CAD build for the part. Positions are in the model's coordinates, mm. Face numbers are marked on the shaded views. A direction names the side the tool comes from. Round coordinates to 2 decimals unless told otherwise and drop trailing zeros. Order: outer loops, then holes, each group sorted by start corner. A loop starts at its lowest first (then second) coordinate and runs counter-clockwise, first axis right, second up. Notation, with made-up numbers: M 75.5,89 L 110.5,89 A25 ccw 110.5,125 Z; hole C 20.25,-34.75 d6. An arc over 180 degrees is marked long. Answer as a JSON object with one key per item and string values.
```python
from build123d import *

# Parameters (mm, degrees)
CYLINDER024_R             = 13
CYLINDER024_DEPTH         = 45
CYLINDER026_R             = 1.95
CYLINDER026_DEPTH         = 10
BOX002_W                  = 21.4
BOX002_H                  = 3.9
BOX002_DEPTH              = 10
FUSION013_PLACEMENT_ANGLE = 90
ARRAY011_COUNT            = 3
CYLINDER028_R             = 2.2
CYLINDER028_DEPTH         = 5
ARRAY013_X_COUNT          = 2
ARRAY013_X_PITCH          = 70
BOX003_W                  = 70
BOX003_H                  = 12
BOX003_DEPTH              = 5
BOX007_W                  = 60
BOX007_H                  = 3
BOX007_DEPTH              = 5
FILLET003_R               = 3
CYLINDER027_R             = 6
CYLINDER027_DEPTH         = 5
ARRAY012_X_COUNT          = 2
ARRAY012_X_PITCH          = 70
CYLINDER025_R             = 16
CYLINDER025_DEPTH         = 45
FUSION016_PLACEMENT_ANGLE = 25
FILLET005_R               = 2


with BuildPart() as internal_cylinder:
    # Cylinder024 → Cylinder024 (new body)
    with BuildSketch(Plane.XY.offset(5)):
        Circle(CYLINDER024_R)
    extrude(amount=CYLINDER024_DEPTH)


with BuildPart() as hole_side001:
    # Cylinder026 → Cylinder026 (new body)
    with BuildSketch(Plane(origin=(21.4, 0, 0), x_dir=(1, 0, 0), z_dir=(0, 0, 1))):
        Circle(CYLINDER026_R)
    extrude(amount=CYLINDER026_DEPTH)


with BuildPart() as middle_hole_fusion:
    # Box002 → Box002 (new body)
    with BuildSketch(Plane(origin=(0, -1.95, 0), x_dir=(1, 0, 0), z_dir=(0, 0, 1))):
        with Locations((10.7, 1.95)):
            Rectangle(BOX002_W, BOX002_H)
    extrude(amount=BOX002_DEPTH)

    # Fusion013: union hole side001
    add(hole_side001.part)


with BuildPart() as middle_hole_fusion_1:
    # Fusion013 placement: moved
    add(middle_hole_fusion.part.moved(Location((-6, 0, 0))).rotate(Axis((-6, 0, 0), (0, -1, 0)), FUSION013_PLACEMENT_ANGLE))

    # Array011: middle hole fusion ×3 about axis
    array011_axis = Axis((0, 0, 0), (0, 0, 1))


with BuildPart() as middle_hole_fusion_2:
    add(middle_hole_fusion_1.part)
    for i in range(1, ARRAY011_COUNT):
        add(middle_hole_fusion_1.part.rotate(array011_axis, i * 360 / ARRAY011_COUNT))


with BuildPart() as middle_hole_fusion_3:
    # Array011 placement: moved
    add(middle_hole_fusion_2.part.moved(Location((0, 0, 5))))

    # Fusion014: union internal cylinder
    add(internal_cylinder.part)


with BuildPart() as spring_plate_end_array001:
    # Cylinder028 → Cylinder028 (new body)
    with BuildSketch(Plane.XY):
        Circle(CYLINDER028_R)
    extrude(amount=CYLINDER028_DEPTH)

    # Array013 X: spring plate end array001 ×2


with BuildPart() as spring_plate_end_array001_1:
    add(spring_plate_end_array001.part)
    with Locations(*[(i * ARRAY013_X_PITCH, 0, 0) for i in range(1, ARRAY013_X_COUNT)]):
        add(spring_plate_end_array001.part)


with BuildPart() as spring_plate_cube:
    # Box003 → Box003 (new body)
    with BuildSketch(Plane(origin=(0, -6, 0), x_dir=(1, 0, 0), z_dir=(0, 0, 1))):
        with Locations((35, 6)):
            Rectangle(BOX003_W, BOX003_H)
    extrude(amount=BOX003_DEPTH)


with BuildPart() as fillet003:
    # Box007 → Box007 (new body)
    with BuildSketch(Plane(origin=(5, -1.5, -5), x_dir=(1, 0, 0), z_dir=(0, 0, 1))):
        with Locations((30, 1.5)):
            Rectangle(BOX007_W, BOX007_H)
    extrude(amount=BOX007_DEPTH)

    # Fillet003
    fillet003_edges = [fillet003.edges().sort_by_distance(p)[0] for p in [
        (5, 0, -5),
        (65, 0, -5),
    ]]
    fillet(fillet003_edges, radius=FILLET003_R)


with BuildPart() as spring_attachment_plate:
    # Cylinder027 → Cylinder027 (new body)
    with BuildSketch(Plane.XY):
        Circle(CYLINDER027_R)
    extrude(amount=CYLINDER027_DEPTH)

    # Array012 X: spring attachment plate ×2


with BuildPart() as spring_attachment_plate_1:
    add(spring_attachment_plate.part)
    with Locations(*[(i * ARRAY012_X_PITCH, 0, 0) for i in range(1, ARRAY012_X_COUNT)]):
        add(spring_attachment_plate.part)

    # Fusion015: union spring plate cube, Fillet003
    add(spring_plate_cube.part)
    add(fillet003.part)

    # Cut009: cut spring plate end array001
    add(spring_plate_end_array001_1.part, mode=Mode.SUBTRACT)


with BuildPart() as spring_attachment_plate_2:
    # Cut009 placement: moved
    add(spring_attachment_plate_1.part.moved(Location((-35, 0, 45))))


with BuildPart() as middle_cut_fillet:
    # Cylinder025 → Cylinder025 (new body)
    with BuildSketch(Plane.XY.offset(5)):
        Circle(CYLINDER025_R)
    extrude(amount=CYLINDER025_DEPTH)

    # Fusion016: union spring attachment plate
    add(spring_attachment_plate_2.part)


with BuildPart() as middle_cut_fillet_1:
    # Fusion016 placement: moved
    add(middle_cut_fillet.part.rotate(Axis((0, 0, 0), (0, 0, 1)), FUSION016_PLACEMENT_ANGLE))

    # Cut008: cut middle hole fusion
    add(middle_hole_fusion_3.part, mode=Mode.SUBTRACT)

    # Fillet005
    fillet005_edges = [middle_cut_fillet_1.edges().sort_by_distance(p)[0] for p in [
        (8.872161, -11.467033, 5),
        (8.872161, 11.467033, 5),
        (5.494662, -13.417033, 5),
        (-14.366823, -1.95, 5),
        (-14.366823, 1.95, 5),
        (5.494662, 13.417033, 5),
    ]]
    fillet(fillet005_edges, radius=FILLET005_R)


solid = middle_cut_fillet_1.part
```
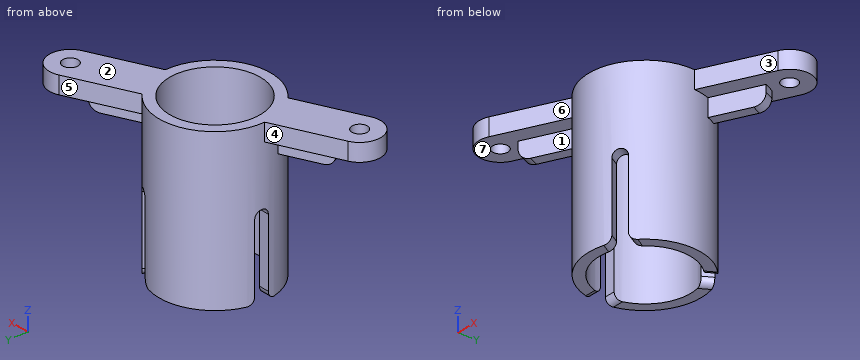
Item 1: Saw through at C-C on x = 0. List the corners of the cut face in (y, z).
Worked answers:
{"outline": "M -16,5 L -13,5 L -13,50 L -16,50 Z; M 13,5 L 16,5 L 16,50 L 13,50 Z"}
Item 2: Saw through at D-D on x = -17.5. List the corners of the cut face in (y, z), and give its area (3 significant figures).
Worked answers:
{"outline": "M -14.78,45 L -9.82,45 L -9.82,40 L -6.51,40 L -6.51,45 L -1.54,45 L -1.54,50 L -14.78,50 Z", "area": "82.8 mm2"}
Item 3: Saw through at B-B on y = 0. List the corners of the cut face in (x, z).
Worked answers:
{"outline": "M -16,28.35 L -13,28.35 L -13,50 L -16,50 Z; M 13,5 L 16,5 L 16,50 L 13,50 Z"}
Item 4: Saw through at A-A on z = 23.5. List the corners of the cut face in (x, y).
Worked answers:
{"outline": "M -15.88,-1.95 A16 ccw 6.25,-14.73 L 4.74,-12.11 A13 cw -12.85,-1.95 Z; M -15.88,1.95 L -12.85,1.95 A13 cw 4.74,12.11 L 6.25,14.73 A16 ccw Z; M 8.12,-10.16 L 9.63,-12.78 A16 ccw 9.63,12.78 L 8.12,10.16 A13 cw Z"}
Item 5: Wall check: line 1 along Y through (x, z) = (0, 38); line 2 along X through (y, z) = (-11, 43.5); line 3 along Z through (x, y) = (-20, -6.5). Give the ranges that are in metal, low to high. Write a range as [from, to].
Worked answers:
{"line 1": "y = [-16, -13], [13, 16]", "line 2": "x = [-27.14, -20.04], [-11.62, -6.93], [6.93, 11.62]", "line 3": "z = [45, 50]"}
Item 6: Drop flat-ended pins along their axis: pin 1 Ø1 at (x, y) = (-15.5, 1) entering from -Z; pin 2 Ø3 at (y, z) = (7, 28) entering from -X (3 decimals); pin 3 Ø3.5 at (x, z) = (-14.5, 13.5) entering from -Y. Give the stop position or say it passes through.
Worked answers:
{"pin 1": "stops at z = 27.65", "pin 2": "stops at x = -15.025", "pin 3": "stops at y = -9.67"}
Item 7: 3-axis set-ups, long thin cutter, end or side, ignore diameter. For the marked faces 4, 5, 6 and 7: which of +Z, -Z, +X, -X, +Y, -Y reach the whole face in a straight line?
Worked answers:
{"face 4": "+Z, -Z, -X, +Y", "face 5": "+Z, -Z, +Y", "face 6": "+Z, -Z, -Y", "face 7": "-Z"}
Item 8: Two-plate mould, pull along X, no slides. Class the marked faces 1, 2 and 3: released by +X, released by -X, zero draft, split by the parting line, or undercut.
Worked answers:
{"face 1": "undercut", "face 2": "zero draft", "face 3": "released by +X"}
